```python
from build123d import *

# Parameters (mm, degrees)
SKETCH1_W           = 177
SKETCH1_H           = 265
SKETCH1_R           = 1.5
BOSS_EXTRUDE1_DEPTH = 5
SKETCH2_W           = 177
SKETCH2_H           = 265
SKETCH2_W_2         = 167.4
SKETCH2_H_2         = 255.4
BOSS_EXTRUDE2_DEPTH = 31.2
FILLET1_R           = 6.82
BOSS_EXTRUDE3_DEPTH = 29.9
SKETCH5_W           = 123
SKETCH5_H           = 5
CUT_EXTRUDE1_DEPTH  = 1.2
SKETCH9_W           = 157.4
SKETCH9_H           = 23.7
CUT_EXTRUDE3_DEPTH  = 10.8
SKETCH10_R          = 2.4
CUT_EXTRUDE4_DEPTH  = 178
SKETCH16_R          = 2.4
CUT_EXTRUDE7_DEPTH  = 177


with BuildPart() as part:
    # Sketch1 → Boss-Extrude1 (new body)
    with BuildSketch(Plane.XY):
        Rectangle(SKETCH1_W, SKETCH1_H)
        with Locations((-57.3, -104.9)):
            Circle(SKETCH1_R, mode=Mode.SUBTRACT)
        with Locations((23.21, -104.9)):
            Circle(SKETCH1_R, mode=Mode.SUBTRACT)
        with Locations((23.21, 104.9)):
            Circle(SKETCH1_R, mode=Mode.SUBTRACT)
        with Locations((-57.3, 104.9)):
            Circle(SKETCH1_R, mode=Mode.SUBTRACT)
    extrude(amount=BOSS_EXTRUDE1_DEPTH)

    # Sketch2 → Boss-Extrude2 (add)
    with BuildSketch(Plane.XY.offset(5)):
        Rectangle(SKETCH2_W, SKETCH2_H)
        Rectangle(SKETCH2_W_2, SKETCH2_H_2, mode=Mode.SUBTRACT)
    extrude(amount=BOSS_EXTRUDE2_DEPTH)

    # Fillet1
    fillet1_edges = [part.edges().sort_by_distance(p)[0] for p in [
        (83.7, -127.7, 20.6),
        (83.7, 127.7, 20.6),
        (-83.7, 127.7, 20.6),
        (-83.7, -127.7, 20.6),
    ]]
    fillet(fillet1_edges, radius=FILLET1_R)

    # Sketch4 → Boss-Extrude3 (add)
    with BuildSketch(Plane.XY.offset(5)):
        with BuildLine():
            Line((83.45267069, -122.7), (-83.45267069, -122.7))
            ThreePointArc((-83.45267069, -122.7), (-81.009164564, -126.307927781), (-76.88, -127.7))
            Line((-76.88, -127.7), (76.88, -127.7))
            ThreePointArc((76.88, -127.7), (81.009164564, -126.307927781), (83.45267069, -122.7))
        make_face()
        with BuildLine():
            ThreePointArc((-76.88, 127.7), (-81.009164564, 126.307927781), (-83.45267069, 122.7))
            Line((-83.45267069, 122.7), (83.45267069, 122.7))
            ThreePointArc((83.45267069, 122.7), (81.009164564, 126.307927781), (76.88, 127.7))
            Line((76.88, 127.7), (-76.88, 127.7))
        make_face()
    extrude(amount=BOSS_EXTRUDE3_DEPTH)

    # Sketch5 → Cut-Extrude1 (cut)
    with BuildSketch(Plane.XY.offset(34.9)):
        with Locations((-14.66, -125.2)):
            Rectangle(SKETCH5_W, SKETCH5_H)
        with Locations((-14.66, 125.2)):
            Rectangle(SKETCH5_W, SKETCH5_H)
    extrude(amount=-CUT_EXTRUDE1_DEPTH, mode=Mode.SUBTRACT)

    # Sketch9 → Cut-Extrude3 (cut, through all)
    with BuildSketch(Plane(origin=(0, -122.7, 0), x_dir=(1, 0, 0), z_dir=(0, 1, 0))):
        with Locations((0, -16.85)):
            Rectangle(SKETCH9_W, SKETCH9_H)
    extrude(amount=-CUT_EXTRUDE3_DEPTH, mode=Mode.SUBTRACT)

    # Sketch10 → Cut-Extrude4 (cut, through all)
    with BuildSketch(Plane(origin=(88.5, 0, 0), x_dir=(0, 0, -1), z_dir=(1, 0, 0))):
        with Locations((-10, -117.5)):
            Circle(SKETCH10_R)
        with Locations((-26.2, -117.5)):
            Circle(SKETCH10_R)
    extrude(amount=-CUT_EXTRUDE4_DEPTH, mode=Mode.SUBTRACT)

    # Sketch16 → Cut-Extrude7 (cut)
    with BuildSketch(Plane(origin=(88.5, 0, 0), x_dir=(0, 0, -1), z_dir=(1, 0, 0))):
        with Locations((-14.5, 117.5)):
            Circle(SKETCH16_R)
        with Locations((-14.5, 87.5)):
            Circle(SKETCH16_R)
        with Locations((-14.5, -52.5)):
            Circle(SKETCH16_R)
        with Locations((-14.5, -82.5)):
            Circle(SKETCH16_R)
    extrude(amount=-CUT_EXTRUDE7_DEPTH, mode=Mode.SUBTRACT)


solid = part.part
```
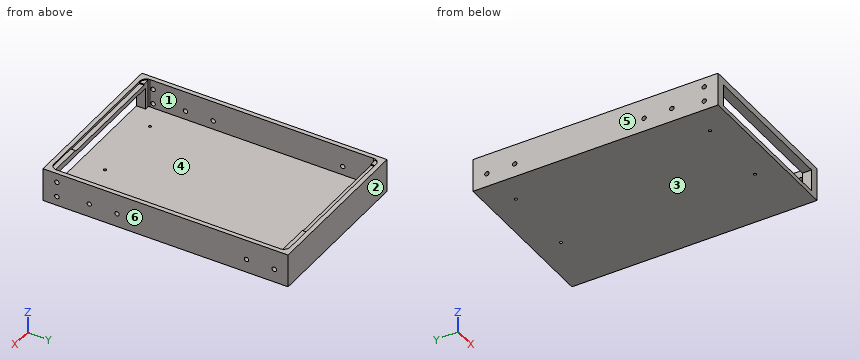
The listing builds one solid part. Answer for the finished solid, in the listing's coordinates (mm). Face numbers are marked on the shaded views. A direction names the side the tool comes from. Round coordinates to 2 decimals unless told otherwise and drop trailing zeros. Order: outer loops, then holes, each group sorted by start corner. A loop starts at its lowest first (then second) coordinate and runs counter-clockwise, first axis right, second up. Notation, with made-up numbers: (-6.75, 59) -> (38.25, 59) arc R28 cw to (38.25, 80) -> close; hole circle Ø10 at (19.25, -16.75). An arc over 180 degrees is marked (long way). Answer as CSV lines item,"result".
Q1. A cutting plane is placed at A-A on x = -64.5. Determine the outline of the cut face in (y, z), plus the area to 3 significant figures.
Computed values:
outline,"(-132.5, 0) -> (132.5, 0) -> (132.5, 36.2) -> (127.7, 36.2) -> (127.7, 33.7) -> (122.7, 33.7) -> (122.7, 5) -> (-132.5, 5) -> close; (-132.5, 28.7) -> (-122.7, 28.7) -> (-122.7, 33.7) -> (-127.7, 33.7) -> (-127.7, 36.2) -> (-132.5, 36.2) -> close"
area,"1,680 mm^2"
Q2. Given pin 1 (2 mm diameter, centred on x = 8.5, y = -25, fed in from -Z); pin 2 (2 mm diameter, centred on x = -5, y = -96.5, fed in from +Z); pin 3 (1.5 mm diameter, centred on x = -31.5, y = -124.5, fed in from +Z); pin 4 (6 mm diameter, centred on x = 23.5, z = 11.5, fed in from -Y), each flat-ended and moving along its own axis, determine where each tip first touches the part or whether it passes through.
Computed values:
pin 1,"stops at z = 0"
pin 2,"stops at z = 5"
pin 3,"stops at z = 33.7"
pin 4,"stops at y = 122.7"
Q3. A cutting plane is placed at B-B on y = -98. Determine the outline of the cut face in (x, z), plus the area to 3 significant figures.
Computed values:
outline,"(-88.5, 0) -> (88.5, 0) -> (88.5, 36.2) -> (83.7, 36.2) -> (83.7, 5) -> (-83.7, 5) -> (-83.7, 36.2) -> (-88.5, 36.2) -> close"
area,"1,180 mm^2"
Q4. For a pull along X with two mould halves and no side action, classify the marked faces 3, 4, 5 and 6 as +X half, -X half, draft (parallel to the pull), parting line (faces both ways), or undercut.
Computed values:
face 3,"draft"
face 4,"undercut"
face 5,"-X half"
face 6,"+X half"
Q5. Consider line 1 (Y direction, x = 87, z = 14); line 2 (Y direction, x = -57.3, z = 2.5); line 3 (X direction, y = -79, z = 29). Determine where each line is inside the solid, lowest interval first. Write a range as from..to.
Computed values:
line 1,"y = -132.5..-84.85, -80.15..-54.85, -50.15..85.15, 89.85..115.15, 119.85..132.5"
line 2,"y = -132.5..-106.4, -103.4..103.4, 106.4..132.5"
line 3,"x = -88.5..-83.7, 83.7..88.5"
Q6. Which of the six approach directions +Z, -Z, +X, -X, +Y, -Y give full straight-line access (tool end or side, diameter ignored) to the marked faces 1 and 2?
Computed values:
face 1,"+Z"
face 2,"+Z, -Z, +X, -X, +Y"
